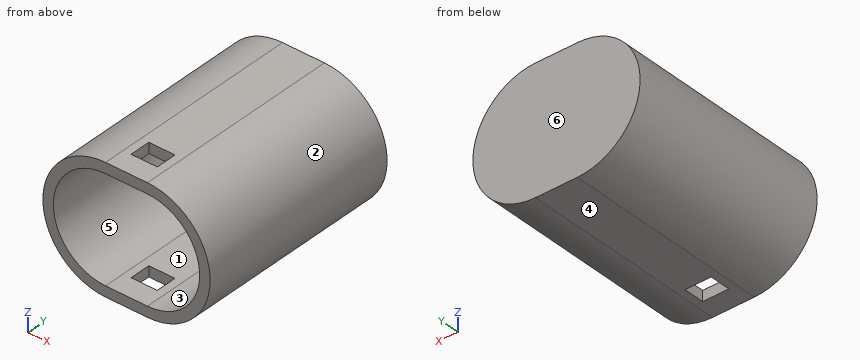
from build123d import *

# Parameters (mm, degrees)
BOSS_EXTRUDE1_DEPTH     = 20
SHELL1_T                = -1
CUT_EXTRUDE1_DEPTH      = 25.657656012
CUT_EXTRUDE1_DEPTH_BACK = 25.657656012
SKETCH2_W               = 2.5
SKETCH2_H               = 2


with BuildPart() as part:
    # Sketch1 → Boss-Extrude1 (new body)
    with BuildSketch(Plane(origin=(0, 0, 0), x_dir=(1, 0, 0), z_dir=(0, 1, 0))):
        with BuildLine():
            Line((-2, -6), (2, -6))
            ThreePointArc((2, -6), (8, 0), (2, 6))
            Line((2, 6), (-2, 6))
            ThreePointArc((-2, 6), (-8, 0), (-2, -6))
        make_face()
    extrude(amount=BOSS_EXTRUDE1_DEPTH)

    # Shell1
    shell1_openings = [part.faces().sort_by_distance(p)[0] for p in [
        (0, 0, 0),
    ]]
    offset(amount=SHELL1_T, openings=shell1_openings, kind=Kind.INTERSECTION)

    # Sketch2 → Cut-Extrude1 (cut, two sides: drawn at the far end of the back side and taken through both)
    with BuildSketch(Plane.XY.offset(6).offset(-CUT_EXTRUDE1_DEPTH_BACK)):
        with Locations((0, 3)):
            Rectangle(SKETCH2_W, SKETCH2_H)
    extrude(amount=CUT_EXTRUDE1_DEPTH + CUT_EXTRUDE1_DEPTH_BACK, mode=Mode.SUBTRACT)


solid = part.part
Geometry: final body of the model. Coordinates: model frame, mm. Face numbers are marked on the shaded views. A direction names the side the tool comes from. Coordinates: 2 decimals unless noted, no trailing zeros. Write each loop counter-clockwise with the first axis right and the second up, starting at its lowest first coordinate (ties: lowest second). Pieces come first, ordered by that corner, then holes. Notation, with made-up numbers: (-39, 24.5) - (-24, 24.5) arc R20 cw to (-24, 41.5) - close; hole circle Ø6 at (8.5, 66.5). An arc over 180 degrees is marked (long way). Return JSON: item names as keys, results as strings.
Item 1: Section query C-C (x = 3.5). Output: boundary loops of the cut face in (y, z).
Completed:
{"outline": "(0, -5.81) - (20, -5.81) - (20, 5.81) - (0, 5.81) - (0, 4.77) - (19, 4.77) - (19, -4.77) - (0, -4.77) - close"}
Item 2: Line query: L1, parallel to Z at x = -6, y = 17.75; L2, parallel to Z at x = -4.25, y = 13.5; L3, parallel to Y at x = -3, z = 2. Output: solid intervals per line, ascending.
Completed:
{"L1": "z = -4.47 to -3, 3 to 4.47", "L2": "z = -5.56 to -4.47, 4.47 to 5.56", "L3": "y = 19 to 20"}
Item 3: Pull-direction query (Z, two-part tool) for the marked faces 1, 2, 3 and 4; classes: +Z half, -Z half, draft (parallel to the pull), parting line (faces both ways), or undercut.
Completed:
{"face 1": "undercut", "face 2": "parting line", "face 3": "undercut", "face 4": "-Z half"}
Item 4: Reachability of the marked faces 5 and 6 from +Z, -Z, +X, -X, +Y, -Y: full face, straight path, thin tool, end or side. Return the list, or none.
Completed:
{"face 5": "-Y", "face 6": "+Z, -Z, +X, -X, +Y"}
Item 5: Pin query (flat end, axial travel): pin 1 Ø3 at (y, z) = (5.5, -3) entering from +X; pin 2 Ø0.5 at (y, z) = (3, 5.5) entering from -X; pin 3 Ø1 at (y, z) = (4, 3) entering from +X. Return the tip coordinate at first contact, or that it passes through.
Completed:
{"pin 1": "stops at x = 7.81", "pin 2": "stops at x = -4.9", "pin 3": "stops at x = 7.45"}
Item 6: Section query B-B (z = 0). Output: boundary loops of the cut face in (x, y).
Completed:
{"outline": "(-8, 0) - (-7, 0) - (-7, 19) - (7, 19) - (7, 0) - (8, 0) - (8, 20) - (-8, 20) - close"}
Item 7: Section query A-A (y = 1.5). Output: boundary loops of the cut face in (x, z), and give its area (3 significant figures).
Completed:
{"outline": "(-2, -6) - (2, -6) arc R6 ccw to (2, 6) - (-2, 6) arc R6 ccw to start; hole (-2, -5) - (2, -5) arc R5 ccw to (2, 5) - (-2, 5) arc R5 ccw to start", "area": "42.6 mm2"}
